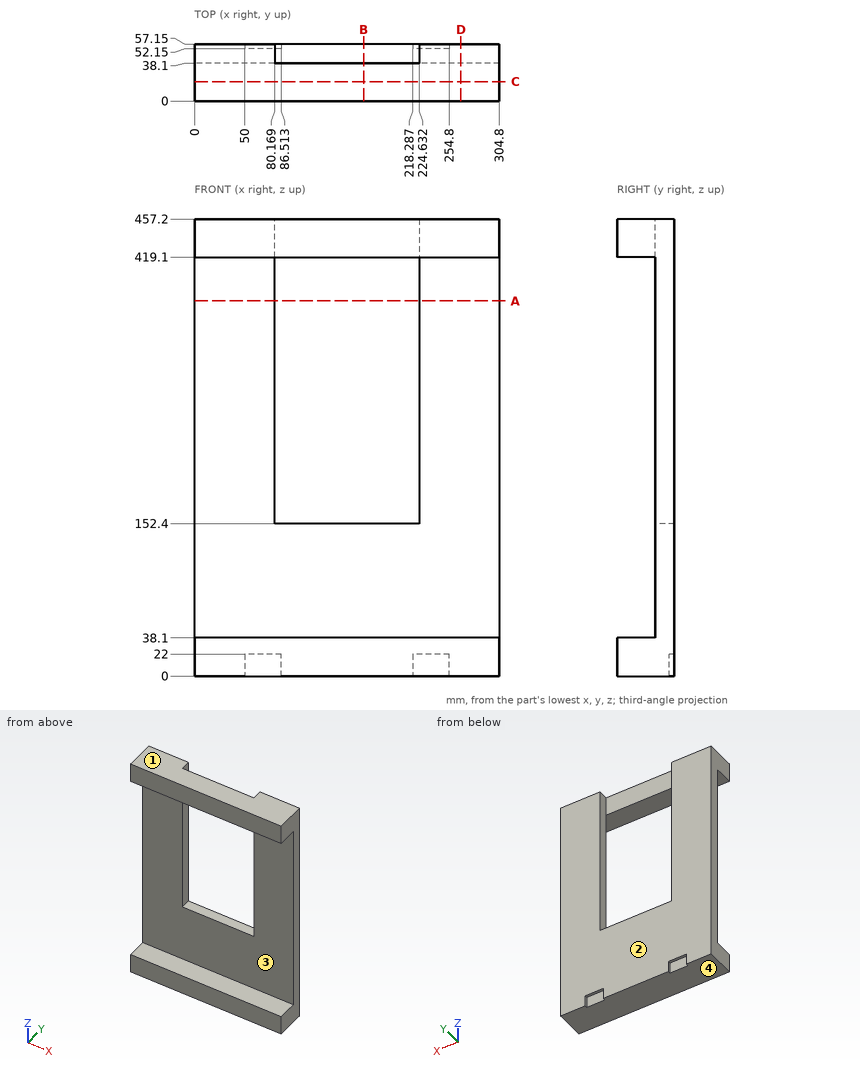
Drawing for the job (mm, zero at the part's lowest x, y, z). Round coordinates to 2 decimals unless told otherwise and drop trailing zeros. Loops run counter-clockwise (first coordinate to the right, second up) from the corner with the lowest first, then second, coordinate; pieces in that order, holes last.
1. Mould opens along Z. For the marked faces 1, 2, 3 and 4 say: +Z half, -Z half, draft (parallel to the pull), parting line (faces both ways), or undercut.
Check values:
face 1: +Z half
face 2: draft
face 3: undercut
face 4: -Z half
2. Band-saw the part on B-B, the plane x = 169. List the corners of the cut face in (y, z).
Check values:
outline: (0, 0) - (57.15, 0) - (57.15, 152.4) - (38.1, 152.4) - (38.1, 38.1) - (0, 38.1) - close; (0, 419.1) - (38.1, 419.1) - (38.1, 457.2) - (0, 457.2) - close
3. Band-saw the part on D-D, the plane x = 266.5. List the corners of the cut face in (y, z).
Check values:
outline: (0, 0) - (57.15, 0) - (57.15, 457.2) - (0, 457.2) - (0, 419.1) - (38.1, 419.1) - (38.1, 38.1) - (0, 38.1) - close
4. Band-saw the part on A-A, the plane z = 375.5. List the corners of the cut face in (x, y), and give its area (3 significant figures).
Check values:
outline: (0, 38.1) - (80.17, 38.1) - (80.17, 57.15) - (0, 57.15) - close; (224.63, 38.1) - (304.8, 38.1) - (304.8, 57.15) - (224.63, 57.15) - close
area: 3,050 mm2
5. Band-saw the part on C-C, the plane y = 19.5. List the corners of the cut face in (x, z), and give its area (3 significant figures).
Check values:
outline: (0, 0) - (304.8, 0) - (304.8, 38.1) - (0, 38.1) - close; (0, 419.1) - (304.8, 419.1) - (304.8, 457.2) - (0, 457.2) - close
area: 23,200 mm2
6. Drop flat-ended pins along their axis: P1, Ø2.5, axis at x = 60.5, y = 53.5, coming from the -Z side; P2, Ø17.5, axis at x = 76, z = 9.5, coming from the +Y side; P3, Ø9.5, axis at x = 182.5, y = 43, coming from the +Z side. Give the stop position or say it passes through.
Check values:
P1: stops at z = 22
P2: stops at y = 52.15
P3: stops at z = 152.4
7. Wall check: probe 1 along X at (y, z) = (50.5, 221.5); probe 2 along Z at (x, y) = (151, 37); probe 3 along Y at (x, z) = (291, 196.5). Give the ranges that are in metal, low to high.
Check values:
probe 1: x = 0 to 80.17, 224.63 to 304.8
probe 2: z = 0 to 38.1, 419.1 to 457.2
probe 3: y = 38.1 to 57.15
